from build123d import *

# Parameters (mm, degrees)
EXTRUDE_1_DEPTH     = 40
SKETCH_2_R          = 2
SKETCH_2_R_2        = 4
CUT_EXTRUDE_1_DEPTH = 40
SKETCH_3_R          = 2
SKETCH_3_R_2        = 4
CUT_EXTRUDE_2_DEPTH = 40
FILLET_1_R          = 3


with BuildPart() as part:
    # Эскиз1 → Бобышка-Вытянуть1 (new body)
    with BuildSketch(Plane.XY):
        with BuildLine():
            Line((-3, 37), (-3, 0))
            ThreePointArc((-3, 0), (-2.121320344, -2.121320344), (0, -3))
            Line((0, -3), (37, -3))
            Line((37, -3), (37, -1))
            Line((37, -1), (0, -1))
            ThreePointArc((0, -1), (-0.707106781, -0.707106781), (-1, 0))
            Line((-1, 0), (-1, 37))
            Line((-1, 37), (-3, 37))
        make_face()
    extrude(amount=EXTRUDE_1_DEPTH)

    # Эскиз2 → Вырез-Вытянуть1 (cut)
    with BuildSketch(Plane.ZY.offset(3)):
        with Locations(Location((7.5, 18.5, 0), (0, 0, 270))):
            Circle(SKETCH_2_R)
        with Locations(Location((20, 31, 0), (0, 0, 270))):
            Circle(SKETCH_2_R)
        with Locations(Location((20, 18.5, 0), (0, 0, 270))):
            Circle(SKETCH_2_R_2)
        with Locations(Location((32.5, 18.5, 0), (0, 0, 270))):
            Circle(SKETCH_2_R)
        with Locations(Location((20, 6, 0), (0, 0, 270))):
            Circle(SKETCH_2_R)
    extrude(amount=-CUT_EXTRUDE_1_DEPTH, mode=Mode.SUBTRACT)

    # Эскиз3 → Вырез-Вытянуть2 (cut)
    with BuildSketch(Plane.XZ.offset(3)):
        with Locations((18.5, 7.5)):
            Circle(SKETCH_3_R)
        with Locations((6, 20)):
            Circle(SKETCH_3_R)
        with Locations((18.5, 32.5)):
            Circle(SKETCH_3_R)
        with Locations((31, 20)):
            Circle(SKETCH_3_R)
        with Locations((18.5, 20)):
            Circle(SKETCH_3_R_2)
    extrude(amount=-CUT_EXTRUDE_2_DEPTH, mode=Mode.SUBTRACT)

    # Скругление1
    fillet_1_edges = [part.edges().sort_by_distance(p)[0] for p in [
        (-2, 37, 0),
        (37, -2, 40),
        (-2, 37, 40),
        (37, -2, 0),
    ]]
    fillet(fillet_1_edges, radius=FILLET_1_R)


solid = part.part
The model under review builds one solid part; all positions refer to its coordinate system, in mm. A direction names the side the tool comes from. Round coordinates to 2 decimals unless told otherwise and drop trailing zeros. Loops run counter-clockwise (first coordinate to the right, second up) from the corner with the lowest first, then second, coordinate; pieces in that order, holes last. Notation, with made-up numbers: (49, 31) -> (59, 31) arc R13 ccw to (59, 49) -> close; hole circle Ø6 at (24, 42.25). An arc over 180 degrees is marked (long way). One line per question, with ' | ' between items. Start each with the question number.
Item 1: For pin 1 (1 mm diameter, centred on y = 27.5, z = 29, fed in from +X); pin 2 (3.5 mm diameter, centred on x = 18.5, z = 32.5, fed in from +Y), all flat-tipped, find the tip position at first contact; note any pin that passes through.
Item 2: Add section D-D, the plane x = 18.5. Write out the cut boundary in (y, z), then the cut area to 3 significant figures.
Item 3: Add section B-B, the plane y = 6. Write out the cut boundary in (x, z).
Item 4: Wall thickness on line 1 along Z through (x, y) = (-1.8, 18.5); line 2 along Z through (x, y) = (18, -2); line 3 along Y through (x, z) = (10, 36.5): over which ranges is each line inside the solid? List them lowest first. Write a range as [from, to].
Item 5: Add section C-C, the plane z = 20. Count the separate pieces of the cut face and the enclosed holes in it, then the cut area to 3 significant figures.
Item 6: Add section A-A, the plane z = 7.5. Write out the cut boundary in (x, y), then the cut area to 3 significant figures.
Item 7: Machinability: for faces 5 (the face through (23, -1, 20)), 6 (the face through (36.1, -1.99, 39.14)), which of the approach directions +Z, -Z, +X, -X, +Y, -Y give a long, thin tool a straight path to every point of the face, cutting with its end or side? Answer none if there is none.
Item 8: Draft analysis for pull direction X (two halves, no side actions). For faces 1 (the face through (-2.14, -2.1, 19.72)), 2 (the face through (-1, 14, 20)), 3 (the face through (17.026, -2.014, 8.852)), 4 (the face through (-2.014, 19.974, 8.852)), state which applies: +X half, -X half, draft (parallel to the pull), parting line (faces both ways), or undercut.
Return value:
1) pin 1: stops at x = -1 | pin 2: passes through
2) outline: (-3, 0) -> (-1, 0) -> (-1, 5.5) -> (-3, 5.5) -> close; (-3, 9.5) -> (-1, 9.5) -> (-1, 16) -> (-3, 16) -> close; (-3, 24) -> (-1, 24) -> (-1, 30.5) -> (-3, 30.5) -> close; (-3, 34.5) -> (-1, 34.5) -> (-1, 40) -> (-3, 40) -> close | area: 48.0 mm2
3) outline: (-3, 0) -> (-1, 0) -> (-1, 18) -> (-3, 18) -> close; (-3, 22) -> (-1, 22) -> (-1, 40) -> (-3, 40) -> close
4) line 1: z = [0, 5.5], [9.5, 16], [24, 30.5], [34.5, 40] | line 2: z = [0, 5.56], [9.44, 16.03], [23.97, 30.56], [34.44, 40] | line 3: y = [-3, -1]
5) separate pieces: 7 | enclosed holes: 0 | area: 90.3 mm2
6) outline: (-3, 0) arc R3 ccw to (0, -3) -> (16.5, -3) -> (16.5, -1) -> (0, -1) arc R1 cw to (-1, 0) -> (-1, 16.5) -> (-3, 16.5) -> close; (-3, 20.5) -> (-1, 20.5) -> (-1, 37) -> (-3, 37) -> close; (20.5, -3) -> (37, -3) -> (37, -1) -> (20.5, -1) -> close | area: 138 mm2
7) face 5: +Z, -Z, +X, +Y | face 6: +Z, +X, +Y, -Y
8) face 1: -X half | face 2: +X half | face 3: undercut | face 4: draft
